```python
from build123d import *

# Parameters (mm, degrees)
BASE_FLANGE1_DEPTH = 2
SKETCH6_W          = 49
SKETCH6_H          = 16.635259071
CUT_EXTRUDE1_DEPTH = 49


# Sheet-metal steps are written as plain solids
with BuildPart() as part:
    # Sketch1 → Base-Flange1 (new body)
    with BuildSketch(Plane(origin=(0, 0, 0), x_dir=(0, 0, -1), z_dir=(1, 0, 0))):
        Polygon((-14.5, -22.025862069), (14.5, -22.025862069), (56.5, 39.324712644), (-56.5, 39.324712644), align=None)
        Polygon((-9.227058078, -12.025862069), (9.227058078, -12.025862069), (37.5352548, 29.324712644), (-37.5352548, 29.324712644), align=None, mode=Mode.SUBTRACT)
    extrude(amount=-BASE_FLANGE1_DEPTH)

    # Sketch6 → Cut-Extrude1 (cut)
    with BuildSketch(Plane(origin=(0, 0, 0), x_dir=(0, 0, -1), z_dir=(1, 0, 0))):
        with Locations((5.5, 37.409748974)):
            Rectangle(SKETCH6_W, SKETCH6_H)
    extrude(amount=-CUT_EXTRUDE1_DEPTH, mode=Mode.SUBTRACT)


solid = part.part
```
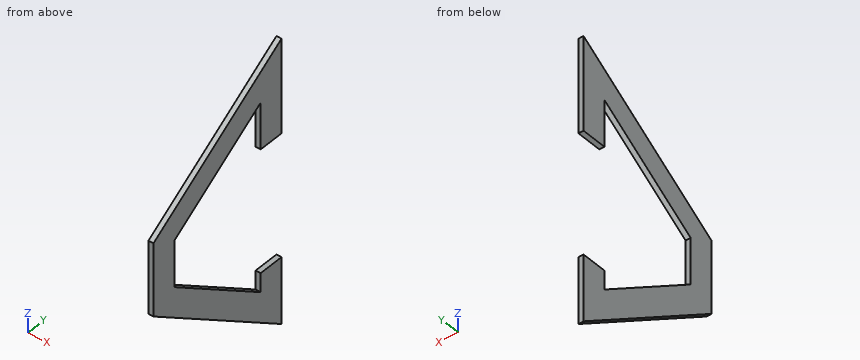
Can you work these out from the model? Positions are in its coordinate system, mm. Give positions to 0.01 mm unless a question says otherwise; leave off trailing zeros. Order: outer loops, then holes, each group sorted by start corner. A loop starts at its lowest first (then second) coordinate and runs counter-clockwise, first axis right, second up. Notation, with made-up numbers: M 32,-13 L 78,-13 A21 cw 78,3 Z; hole C -35.5,57.5 d10. An arc over 180 degrees is marked long. Write item = value, one per line. Start each with the question number.
Q1. Will these pins go through, and if not, where does the flat tip stop? pin 1 Ø12 at (y, z) = (4, -43) entering from +X; pin 2 Ø1 at (x, y) = (-0.5, 34.5) entering from -Z; pin 3 Ø1 at (x, y) = (-1, 1.5) entering from +Z; pin 4 Ø0.6 at (x, y) = (-1, 35) entering from +Z.
Q2. Suppose I cut it at B-B (x = -1.2). Write out the boundary of the cut face in (y, z).
Q3. Suppose I cut it at A-A (y = 26). Write out the boundary of the cut face in (x, z).
Q4. I need wall thicknesses on probe 1 along Z at (x, y) = (-0.2, 7.5); probe 2 along Z at (x, y) = (-1.65, -3); probe 3 along Y at (x, z) = (-1.55, 27.5). Which ranges of each line are inside material? Lowest first, please. Write a range as [from, to].
Q5. Suppose I cut it at D-D (z = -23.5). Write out the boundary of the cut face in (x, y).
Q6. Suppose I cut it at C-C (z = 23.5). Write out the boundary of the cut face in (x, y).
Check result:
q1.pin_1 = through
q1.pin_2 = -53.54
q1.pin_3 = 30.95
q1.pin_4 = 53.74
q2.outline = M -22.03,-14.5 L 39.32,-56.5 L 39.32,-30 L 29.32,-30 L 29.32,-37.54 L -12.03,-9.23 L -12.03,9.23 L 29.32,37.54 L 29.32,19 L 39.32,19 L 39.32,56.5 L -22.03,14.5 Z
q3.outline = M -2,-47.38 L 0,-47.38 L 0,-35.26 L -2,-35.26 Z; M -2,35.26 L 0,35.26 L 0,47.38 L -2,47.38 Z
q4.probe_1 = [-34.71, -22.59], [22.59, 34.71]
q4.probe_2 = [-27.52, -15.41], [15.41, 27.52]
q4.probe_3 = [-3.04, 14.67], [29.32, 39.32]
q5.outline = M -2,-8.88 L 0,-8.88 L 0,8.82 L -2,8.82 Z
q6.outline = M -2,-8.88 L 0,-8.88 L 0,8.82 L -2,8.82 Z; M -2,29.32 L 0,29.32 L 0,39.32 L -2,39.32 Z
